```python
from build123d import *

# Parameters (mm, degrees)
F0_W        = 142.875
F0_H        = 9.525
F1_DEPTH    = 12.7
F3_DEPTH    = 142.875
F5_DEPTH    = 9.525
F6_DEPTH    = 142.875
F7_T1_DEPTH = 101.5751710417
F7_T3_DEPTH = 45.552419836
F7_T5_DEPTH = 139.7
F8_R        = 5.08
F9_DEPTH    = 60.325


# Not quite as in the source:
# - a fillet or chamfer that OpenCascade refuses, or shapes differently, is made with other operations: its cross-section is extruded or revolved along the edge and cut away or added


with BuildPart() as f1:
    # F0 (on Front) → F1 (new body, symmetric)
    with BuildSketch(Plane.XZ):
        Polygon((-20.4177256674, 25.4), (-83.9177256674, 25.4), (-83.9177256674, 0), (30.3822743326, 0), (30.3822743326, 6.35), (43.0822743326, 6.35), (48.3298544966, 0), (68.4822743326, 0), (68.4822743326, 7.9375), (-74.3927256674, 7.9375), (-74.3927256674, 17.4625), (68.4822743326, 17.4625), (68.4822743326, 22.225), (-20.4177256674, 22.225), align=None)
        with Locations((-2.9552256674, 12.7)):
            Rectangle(F0_W, F0_H)
    extrude(amount=F1_DEPTH, both=True)

    # F2 (on face) → F3 (cut)
    with BuildSketch(Plane.YZ.offset(68.4822743326)):
        with BuildLine():
            Line((-4.7625, 12.7), (0, 12.7))
            Line((0, 12.7), (4.7625, 12.7))
            ThreePointArc((4.7625, 12.7), (0, 17.4625), (-4.7625, 12.7))
        make_face()
        with BuildLine():
            Line((-1.5875, 8.2098719395), (0, 8.2098719395))
            Line((0, 8.2098719395), (0, 12.7))
            Line((0, 12.7), (-4.7625, 12.7))
            ThreePointArc((-4.7625, 12.7), (-3.8885649667, 9.950369343), (-1.5875, 8.2098719395))
        make_face()
        with BuildLine():
            ThreePointArc((-1.5875, 8.2098719395), (-0.8053481737, 8.0060868597), (0, 7.9375))
            Line((0, 7.9375), (0, 8.2098719395))
            Line((0, 8.2098719395), (-1.5875, 8.2098719395))
        make_face()
        with BuildLine():
            Line((0, 8.2098719395), (0, 7.9375))
            ThreePointArc((0, 7.9375), (0.8053481737, 8.0060868597), (1.5875, 8.2098719395))
            Line((1.5875, 8.2098719395), (0, 8.2098719395))
        make_face()
        with BuildLine():
            Line((0, 12.7), (0, 8.2098719395))
            Line((0, 8.2098719395), (1.5875, 8.2098719395))
            ThreePointArc((1.5875, 8.2098719395), (3.8885649667, 9.950369343), (4.7625, 12.7))
            Line((4.7625, 12.7), (0, 12.7))
        make_face()
    extrude(amount=-F3_DEPTH, mode=Mode.SUBTRACT)

    # F4 (on face) → F5 (cut)
    with BuildSketch(Plane(origin=(-83.9177256674, 0, 0), x_dir=(0, -1, 0), z_dir=(-1, 0, 0))):
        with BuildLine():
            Line((-0.79375, 12.7), (0.79375, 12.7))
            ThreePointArc((0.79375, 12.7), (0, 13.49375), (-0.79375, 12.7))
        make_face()
        with BuildLine():
            ThreePointArc((-0.79375, 12.7), (0, 11.90625), (0.79375, 12.7))
            Line((0.79375, 12.7), (-0.79375, 12.7))
        make_face()
    extrude(amount=-F5_DEPTH, mode=Mode.SUBTRACT)

    # F2 (on face) → F6 (cut)
    with BuildSketch(Plane.YZ.offset(68.4822743326)):
        with BuildLine():
            ThreePointArc((12.7, 17.4625), (9.3324039546, 16.0675960454), (7.9375, 12.7))
            Line((7.9375, 12.7), (12.7, 12.7))
            Line((12.7, 12.7), (12.7, 17.4625))
        make_face()
        with BuildLine():
            ThreePointArc((7.9375, 12.7), (9.3324039546, 9.3324039546), (12.7, 7.9375))
            Line((12.7, 7.9375), (12.7, 12.7))
            Line((12.7, 12.7), (7.9375, 12.7))
        make_face()
        with BuildLine():
            Line((-12.7, 12.7), (-12.7, 7.9375))
            ThreePointArc((-12.7, 7.9375), (-9.3324039546, 9.3324039546), (-7.9375, 12.7))
            Line((-7.9375, 12.7), (-12.7, 12.7))
        make_face()
        with BuildLine():
            Line((-12.7, 12.7), (-7.9375, 12.7))
            ThreePointArc((-7.9375, 12.7), (-9.3324039546, 16.0675960454), (-12.7, 17.4625))
            Line((-12.7, 17.4625), (-12.7, 12.7))
        make_face()
    extrude(amount=-F6_DEPTH, mode=Mode.SUBTRACT)

    # F7: fillet of radius 5.08 on 6 edges, made by hand

    # F7_s2 → F7_t1 (cut)
    with BuildSketch(Plane.YZ.offset(-20.4177256674)):
        with BuildLine():
            ThreePointArc((7.6299315833, 22.225), (11.1079698235, 20.8476544532), (12.7, 17.4625))
            Line((12.7, 17.4625), (12.7, 22.225))
            Line((12.7, 22.225), (7.6299315833, 22.225))
        make_face()
        with BuildLine():
            ThreePointArc((-7.6299315833, 22.225), (-11.1079698235, 20.8476544532), (-12.7, 17.4625))
            Line((-12.7, 17.4625), (-12.7, 22.225))
            Line((-12.7, 22.225), (-7.6299315833, 22.225))
        make_face()
    extrude(amount=F7_T1_DEPTH, mode=Mode.SUBTRACT)

    # F7_s4 → F7_t3 (cut)
    with BuildSketch(Plane.YZ.offset(35.6298544966)):
        with BuildLine():
            ThreePointArc((12.7, 5.08), (11.2121024484, 1.4878975516), (7.62, 0))
            Line((7.62, 0), (12.7, 0))
            Line((12.7, 0), (12.7, 5.08))
        make_face()
        with BuildLine():
            ThreePointArc((-12.7, 5.08), (-11.2121024484, 1.4878975516), (-7.62, 0))
            Line((-7.62, 0), (-12.7, 0))
            Line((-12.7, 0), (-12.7, 5.08))
        make_face()
    extrude(amount=F7_T3_DEPTH, mode=Mode.SUBTRACT)

    # F7_s6 → F7_t5 (cut)
    with BuildSketch(Plane.YZ.offset(-96.6177256674)):
        with BuildLine():
            ThreePointArc((-12.7, 5.08), (-11.2121024484, 1.4878975516), (-7.62, 0))
            Line((-7.62, 0), (-12.7, 0))
            Line((-12.7, 0), (-12.7, 5.08))
        make_face()
        with BuildLine():
            ThreePointArc((12.7, 5.08), (11.2121024484, 1.4878975516), (7.62, 0))
            Line((7.62, 0), (12.7, 0))
            Line((12.7, 0), (12.7, 5.08))
        make_face()
    extrude(amount=F7_T5_DEPTH, mode=Mode.SUBTRACT)

    # F8
    f8_edges = [f1.edges().sort_by_distance(p)[0] for p in [
        (-52.167726, 12.7, 25.4),
        (-52.167726, -12.7, 25.4),
    ]]
    fillet(f8_edges, radius=F8_R)

    # F2 (on face) → F9 (cut)
    with BuildSketch(Plane.YZ.offset(68.4822743326)):
        with BuildLine():
            Line((0, 7.9375), (0, 0))
            Line((0, 0), (1.5875, 0))
            Line((1.5875, 0), (1.5875, 8.2098719395))
            ThreePointArc((1.5875, 8.2098719395), (0.8053481737, 8.0060868597), (0, 7.9375))
        make_face()
        with BuildLine():
            Line((-1.5875, 0), (0, 0))
            Line((0, 0), (0, 7.9375))
            ThreePointArc((0, 7.9375), (-0.8053481737, 8.0060868597), (-1.5875, 8.2098719395))
            Line((-1.5875, 8.2098719395), (-1.5875, 0))
        make_face()
    extrude(amount=-F9_DEPTH, mode=Mode.SUBTRACT)


solid = f1.part
```
Work out the finished part from the listing and answer in its coordinate system (mm). A direction names the side the tool comes from. Coordinates: 2 decimals unless noted, no trailing zeros. Loops run counter-clockwise (first coordinate to the right, second up) from the corner with the lowest first, then second, coordinate; pieces in that order, holes last. Notation, with made-up numbers: M 47.5,25 L 69.5,25 A14 cw 69.5,32 Z; hole C 26.5,83.25 d6. An arc over 180 degrees is marked long. Use CSV: the item, a comma, the result in double quotes. Start each with the question number.
(1) Find section A-A, the plane x = -47.5. Give the vertices of the cut face in (y, z) (1 decimal).
(2) For a pull along X with two mould halves and no side action, classify faces 1 (the face through (-83.918, 0, 10)), 2 (the face through (-25.7, -12.7, 7.7)), 3 (the face through (30.382, 7, 3)), 4 (the face through (37, 7, 6.35)) as +X half, -X half, draft (parallel to the pull), parting line (faces both ways), or undercut.
(3) Consider line 1 (Y direction, x = -78, z = 12.7); line 2 (Z direction, x = -77, y = 0); line 3 (X direction, y = -9, z = 10.5). Determine where each line is inside the solid, lowest interval first.
(4) Given pin 1 Ø5.5 at (x, y) = (37, -6.5) entering from -Z; pin 2 Ø7.5 at (x, y) = (8, 0) entering from +Z (3 decimals); pin 3 Ø5 at (y, z) = (-11, 11.5) entering from +X; pin 4 Ø1 at (y, z) = (0, 12.7) entering from -X, each flat-ended and moving along its own axis, determine where each tip first touches the part or whether it passes through.
(5) Find section C-C, the plane y = -9.5. Give the vertices of the cut face in (x, z).
(6) Find section D-D, the plane z = 15.5. Give the vertices of the cut face in (x, y), then the cut area to 3 significant figures.
(7) For faces 5 (the face through (23.41, -11.069, 20.884)), 6 (the face through (45.67, 7.07, 3.22)), 7 (the face through (39, 1.588, 7)), 8 (the face through (-74.393, -11, 13)), determine the directions among +Z, -Z, +X, -X, +Y, -Y from which every point of the face is accessible in a straight line to the end or side of a thin tool.
Recorded:
1,outline,"M -12.7,5.1 A5.1 ccw -7.6,0 L 7.6,0 A5.1 ccw 12.7,5.1 L 12.7,7.9 A4.8 cw 12.7,17.5 L 12.7,20.3 A5.1 ccw 7.6,25.4 L -7.6,25.4 A5.1 ccw -12.7,20.3 L -12.7,17.5 A4.8 cw -12.7,7.9 Z; hole C 0,12.7 d9.5"
2,face 1,"-X half"
2,face 2,"draft"
2,face 3,"undercut"
2,face 4,"undercut"
3,line 1,"y = -12.7 to -0.79, 0.79 to 12.7"
3,line 2,"z = 0 to 11.91, 13.49 to 25.4"
3,line 3,"x = -83.92 to -74.39"
4,pin 1,"stops at z = 6.35"
4,pin 2,"stops at z = 22.225"
4,pin 3,"stops at x = -74.39"
4,pin 4,"passes through"
5,outline,"M -83.92,0.36 L 30.38,0.36 L 30.38,6.35 L 43.08,6.35 L 48.03,0.36 L 68.48,0.36 L 68.48,9.17 L -74.39,9.17 L -74.39,16.23 L 68.48,16.23 L 68.48,21.87 L -20.42,21.87 L -20.42,25.04 L -83.92,25.04 Z"
6,outline,"M -83.92,-12.7 L -74.39,-12.7 L -74.39,-8.85 L 68.48,-8.85 L 68.48,-3.85 L -74.39,-3.85 L -74.39,3.85 L 68.48,3.85 L 68.48,8.85 L -74.39,8.85 L -74.39,12.7 L -83.92,12.7 Z"
6,area,"1,670 mm^2"
7,face 5,"+Z, +X, -Y"
7,face 6,"-Z, +Y, -Y"
7,face 7,"-Z, +X"
7,face 8,"+X, -Y"
